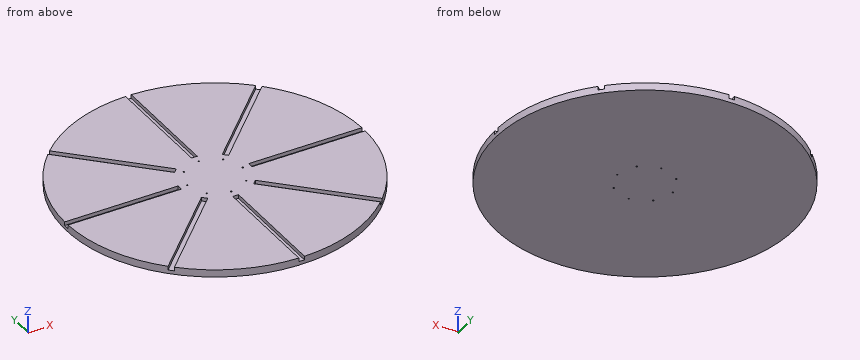
from build123d import *

# Parameters (mm, degrees)
F0_R      = 400
F1_DEPTH  = 20
F3_R      = 2
F4_DEPTH  = 20
F5_R      = 2
F6_DEPTH  = 20
F8_R      = 2
F9_DEPTH  = 20
F10_R     = 2
F11_DEPTH = 20
F12_R     = 2
F13_DEPTH = 20
F14_R     = 2
F15_DEPTH = 20
F16_R     = 1.4677946232
F17_DEPTH = 20
F18_R     = 2
F19_DEPTH = 20
F20_W     = 15.2905675913
F20_H     = 305
F20_W_2   = 305
F20_H_2   = 15.2905675913
F21_DEPTH = 10


with BuildPart() as f1:
    # F0 (on Top) → F1 (new body)
    with BuildSketch(Plane.XY):
        Circle(F0_R)
    extrude(amount=-F1_DEPTH)

    # F3 (on Top) → F4 (cut)
    with BuildSketch(Plane.XY):
        with Locations((-75, 0)):
            Circle(F3_R)
    extrude(amount=-F4_DEPTH, mode=Mode.SUBTRACT)

    # F5 (on Top) → F6 (cut)
    with BuildSketch(Plane.XY):
        with Locations((-53.1572374294, -52.9084880607)):
            Circle(F5_R)
    extrude(amount=-F6_DEPTH, mode=Mode.SUBTRACT)

    # F8 (on offset) → F9 (cut)
    with BuildSketch(Plane.XY):
        with Locations((0, -75)):
            Circle(F8_R)
    extrude(amount=-F9_DEPTH, mode=Mode.SUBTRACT)

    # F10 (on offset) → F11 (cut)
    with BuildSketch(Plane.XY):
        with Locations((53.3727891743, -52.9747456312)):
            Circle(F10_R)
    extrude(amount=-F11_DEPTH, mode=Mode.SUBTRACT)

    # F12 (on offset) → F13 (cut)
    with BuildSketch(Plane.XY):
        with Locations((75, 0)):
            Circle(F12_R)
    extrude(amount=-F13_DEPTH, mode=Mode.SUBTRACT)

    # F14 (on offset) → F15 (cut)
    with BuildSketch(Plane.XY):
        with Locations((53.0946776271, 53.1038790941)):
            Circle(F14_R)
    extrude(amount=-F15_DEPTH, mode=Mode.SUBTRACT)

    # F16 (on offset) → F17 (cut)
    with BuildSketch(Plane.XY):
        with Locations((0, 75)):
            Circle(F16_R)
    extrude(amount=-F17_DEPTH, mode=Mode.SUBTRACT)

    # F18 (on offset) → F19 (cut)
    with BuildSketch(Plane.XY):
        with Locations((-53.0560910702, 53.0486702919)):
            Circle(F18_R)
    extrude(amount=-F19_DEPTH, mode=Mode.SUBTRACT)

    # F20 (on offset) → F21 (cut)
    with BuildSketch(Plane.XY):
        with Locations((0, -247.5)):
            Rectangle(F20_W, F20_H)
        Polygon((288.2487444906, -277.4366804586), (72.5811762287, -61.7691121967), (61.7691121967, -72.5811762287), (277.4366804586, -288.2487444906), align=None)
        with Locations((247.5, 0)):
            Rectangle(F20_W_2, F20_H_2)
        Polygon((277.4366804586, 288.2487444906), (61.7691121967, 72.5811762287), (72.5811762287, 61.7691121967), (288.2487444906, 277.4366804586), align=None)
        with Locations((0, 247.5)):
            Rectangle(F20_W, F20_H)
        Polygon((-288.2487444906, 277.4366804586), (-72.5811762287, 61.7691121967), (-61.7691121967, 72.5811762287), (-277.4366804586, 288.2487444906), align=None)
        with Locations((-247.5, 0)):
            Rectangle(F20_W_2, F20_H_2)
        Polygon((-277.4366804586, -288.2487444906), (-61.7691121967, -72.5811762287), (-72.5811762287, -61.7691121967), (-288.2487444906, -277.4366804586), align=None)
    extrude(amount=-F21_DEPTH, mode=Mode.SUBTRACT)


solid = f1.part
Build history of the part. All positions in model axes, mm. Round coordinates to 2 decimals unless told otherwise and drop trailing zeros. Order: outer loops, then holes, each group sorted by start corner. A loop starts at its lowest first (then second) coordinate and runs counter-clockwise, first axis right, second up. Notation, with made-up numbers: M -39,-1 L -24,-1 A25 ccw -24,31 Z; hole C 73,-33.75 d4. An arc over 180 degrees is marked long. Use CSV: the item, a comma, the result in double quotes. Start each with the question number.
(1) Cut at A-A on y = -257.5. List the corners of the cut face in (x, z), then the cut area to 3 significant figures.
(2) Cut at C-C on z = -16.25. State how many separate pieces and enclosed holes the cut face has, then the cut area to 3 significant figures.
(3) Cut at D-D on x = -339.5. List the corners of the cut face in (y, z).
(4) Cut at B-B on x = 123. List the corners of the cut face in (y, z).
(5) Drill centre lines: probe 1 along Y at (x, z) = (164.5, -1.75); probe 2 along Y at (x, z) = (252.5, -9); probe 3 along X at (y, z) = (-110.5, -1.5). Where is each one in solid material? Low to high.
(6) Flat gauge pins, fed straight in: P1, Ø5, axis at y = -206, z = -3, coming from the -X side; P2, Ø2.5, axis at x = 0, y = 75, coming from the -Z side; P3, Ø2, axis at x = -85, z = -16.5, coming from the -Y side; P4, Ø5, axis at x = -260.5, z = -9, coming from the +Y side. Where does each tip first touch, or does it go through?
Findings:
1,outline,"M -306.09,-20 L 306.09,-20 L 306.09,0 L 268.31,0 L 268.31,-10 L 246.69,-10 L 246.69,0 L 7.65,0 L 7.65,-10 L -7.65,-10 L -7.65,0 L -246.69,0 L -246.69,-10 L -268.31,-10 L -268.31,0 L -306.09,0 Z"
1,area,"11,700 mm^2"
2,separate pieces,"1"
2,enclosed holes,"8"
2,area,"503,000 mm^2"
3,outline,"M -211.52,-20 L 211.52,-20 L 211.52,0 L 7.65,0 L 7.65,-10 L -7.65,-10 L -7.65,0 L -211.52,0 Z"
4,outline,"M -380.62,-20 L 380.62,-20 L 380.62,0 L 133.81,0 L 133.81,-10 L 112.19,-10 L 112.19,0 L 7.65,0 L 7.65,-10 L -7.65,-10 L -7.65,0 L -112.19,0 L -112.19,-10 L -133.81,-10 L -133.81,0 L -380.62,0 Z"
5,probe 1,"y = -364.61 to -175.31, -153.69 to -7.65, 7.65 to 153.69, 175.31 to 364.61"
5,probe 2,"y = -310.23 to -263.31, -241.69 to -7.65, 7.65 to 241.69, 263.31 to 310.23"
5,probe 3,"x = -384.43 to -121.31, -99.69 to -7.65, 7.65 to 99.69, 121.31 to 384.43"
6,P1,"stops at x = -344.37"
6,P2,"passes through"
6,P3,"stops at y = -391.08"
6,P4,"stops at y = 305.67"
